Here's how the part is built. I have some questions about the finished solid (model axes, mm). A direction names the side the tool comes from. Round coordinates to 2 decimals unless told otherwise and drop trailing zeros. Loops run counter-clockwise (first coordinate to the right, second up) from the corner with the lowest first, then second, coordinate; pieces in that order, holes last. Notation, with made-up numbers: (-40, -21.75) - (-25, -21.75) arc R30 ccw to (-25, 10.25) - close; hole circle Ø11 at (-14, 7). An arc over 180 degrees is marked (long way). Answer as a JSON object with one key per item and string values. Group by question number.
1) I want a section at C-C, the plane x = 30. Please give me the cut outline in (y, z).
2) I want a section at D-D, the plane z = 46. Please give me the cut outline in (x, y), then the cut area to 3 significant figures.
3) I want a section at B-B, the plane y = 21.75. Please give me the cut outline in (x, z), then the cut area to 3 significant figures.
4) If I drill on line 1 along Z through (x, y) = (27.5, 21.75); line 2 along Z through (x, y) = (14.5, 7.75); line 3 along Z through (x, y) = (18.5, 21.75), over which ranges is the centre line in solid material (lowest first)? Write a range as [from, to].
5) I want a section at A-A, the plane y = 12. Give the number of separate pieces and of enclosed holes in the cut face, then the cut area to 3 significant figures.
6) If we mould it in two halves opening along Z, with no side actions, what happens to faces 1 (the face through (30, 12, 0)), 2 (the face through (21.584, 11.832, 27.473)), 3 (the face through (4.289, 11.832, 58.196))? For each: pulls with the +Z half, pulls with the -Z half, needs draft (parallel to the pull), parting line crosses it, or undercut.
7) Which directions (+Z, -Z, +X, -X, +Y, -Y) give clear straight access to the entire face, cutting with the end or side of a thin tool? Please do faces 4 (the face through (27.453, 11.832, 21.604)), 5 (the face through (29.8, 11.83, 17.78)), 6 (the face through (8.58, 11.83, 29.87)), 7 (the face through (2.96, 12.46, 48.47)).
8) Will these pins go through, and if not, where does the flat tip stop? P1, Ø8, axis at y = 5, z = 39, coming from the +X side; P2, Ø6.5, axis at x = 40.5, y = 17.5, coming from the +Z side; P3, Ø3, axis at y = 11, z = 22.5, coming from the +X side.
from build123d import *

# Parameters (mm, degrees)
F1_DEPTH = 24
F2_R     = 3.5
F3_DEPTH = 6
F4_R     = 3.5
F5_DEPTH = 6


# Not quite as in the source:
# - ends of sketch curves that miss each other by under 0.0002 mm in the source are joined


with BuildPart() as f1:
    # F0 (on Front) → F1 (new body)
    with BuildSketch(Plane.XZ):
        with BuildLine():
            Line((5.999886, 45.000227), (-0.000114, 45.000227))
            Line((-0.000114, 45.000227), (-0.000114, 0.000227))
            Line((-0.000114, 0.000227), (44.999886, 0.000227))
            Line((44.999886, 0.000227), (44.999886, 6.000227))
            Line((44.999886, 6.000227), (32.449634, 6.000227))
            Line((32.449634, 6.000227), (27.356487, 11.093373))
            ThreePointArc((27.356487, 11.093373), (26.477808, 13.214693), (27.3564876564, 15.3360133436))
            Line((27.3564876564, 15.3360133436), (32.306235, 20.285761))
            Line((32.306235, 20.285761), (28.523214, 24.068783))
            Line((28.523214, 24.068783), (26.755447, 22.301016))
            Line((26.755447, 22.301016), (28.16966, 20.886802))
            Line((28.16966, 20.886802), (23.960753, 16.677895))
            Line((23.960753, 16.677895), (16.64382, 21.098934))
            Line((16.64382, 21.098934), (18.091767, 22.546881))
            Line((18.091767, 22.546881), (16.677553, 23.961095))
            Line((16.677553, 23.961095), (20.88646, 28.170002))
            Line((20.88646, 28.170002), (22.300674, 26.755788))
            Line((22.300674, 26.755788), (24.068441, 28.523555))
            Line((24.068441, 28.523555), (20.28542, 32.306577))
            Line((20.28542, 32.306577), (15.335672, 27.356829))
            ThreePointArc((15.335672, 27.356829), (13.2143523536, 26.47815), (11.0930316564, 27.3568296564))
            Line((11.0930316564, 27.3568296564), (5.999886, 32.449975))
            Line((5.999886, 32.449975), (5.999886, 45.000227))
        make_face()
        with BuildLine():
            ThreePointArc((4.499886, 4.000227), (4.1463326094, 4.1466736094), (3.999886, 4.500227))
            Line((3.999886, 4.500227), (3.999886, 29.000227))
            ThreePointArc((3.999886, 29.000227), (4.3085446105, 29.4621669016), (4.8534398906, 29.3537798906))
            Line((4.8534398906, 29.3537798906), (13.567905, 20.639315))
            Line((13.567905, 20.639315), (11.243789, 18.315199))
            ThreePointArc((11.243789, 18.315199), (10.3880809238, 17.170688427), (9.8910739732, 15.8308650058))
            Line((9.8910739732, 15.8308650058), (11.753138, 13.968801))
            Line((11.753138, 13.968801), (12.364509, 14.132617))
            ThreePointArc((12.364509, 14.132617), (16.54708952, 16.547432386), (14.1322760675, 12.364850252))
            Line((14.1322760675, 12.364850252), (13.968459, 11.75348))
            Line((13.968459, 11.75348), (15.830523, 9.891416))
            ThreePointArc((15.830523, 9.891416), (17.1703461165, 10.3884227548), (18.3148569059, 11.2441310941))
            Line((18.3148569059, 11.2441310941), (20.638973, 13.568247))
            Line((20.638973, 13.568247), (29.353439, 4.853781))
            ThreePointArc((29.353439, 4.853781), (29.461825631, 4.3088849572), (28.999886, 4.000227))
            Line((28.999886, 4.000227), (4.499886, 4.000227))
        make_face(mode=Mode.SUBTRACT)
        with BuildLine():
            Line((3.999886, 29.000227), (3.999886, 4.500227))
            ThreePointArc((3.999886, 4.500227), (4.1463326094, 4.1466736094), (4.499886, 4.000227))
            Line((4.499886, 4.000227), (28.999886, 4.000227))
            ThreePointArc((28.999886, 4.000227), (29.461825631, 4.3088849572), (29.3534398906, 4.8537798906))
            Line((29.3534398906, 4.8537798906), (20.638973, 13.568247))
            Line((20.638973, 13.568247), (18.314857, 11.244131))
            ThreePointArc((18.314857, 11.244131), (17.1703461165, 10.3884227548), (15.8305230058, 9.8914159732))
            Line((15.8305230058, 9.8914159732), (13.968459, 11.75348))
            Line((13.968459, 11.75348), (14.132276, 12.36485))
            ThreePointArc((14.132276, 12.36485), (16.54708952, 16.547432386), (12.364508569, 14.1326168845))
            Line((12.364508569, 14.1326168845), (11.753138, 13.968801))
            Line((11.753138, 13.968801), (9.891074, 15.830865))
            ThreePointArc((9.891074, 15.830865), (10.3880809238, 17.170688427), (11.2437895941, 18.3151994059))
            Line((11.2437895941, 18.3151994059), (13.567905, 20.639315))
            Line((13.567905, 20.639315), (4.853439, 29.353781))
            ThreePointArc((4.853439, 29.353781), (4.3085446105, 29.4621669016), (3.999886, 29.000227))
        make_face()
        with BuildLine():
            ThreePointArc((5.999886, 54.000227), (4.2425266871, 58.2428676871), (-0.000114, 60.000227))
            Line((-0.000114, 60.000227), (-0.000114, 45.000227))
            Line((-0.000114, 45.000227), (5.999886, 45.000227))
            Line((5.999886, 45.000227), (5.999886, 54.000227))
        make_face()
        with BuildLine():
            Line((44.999886, 6.000227), (44.999886, 0.000227))
            Line((44.999886, 0.000227), (59.999886, 0.000227))
            ThreePointArc((59.999886, 0.000227), (58.2425266871, 4.2428676871), (53.999886, 6.000227))
            Line((53.999886, 6.000227), (44.999886, 6.000227))
        make_face()
    extrude(amount=-F1_DEPTH)

    # F2 (on face) → F3 (cut)
    with BuildSketch(Plane(origin=(-0.000114, 0, 0), x_dir=(0, -1, 0), z_dir=(-1, 0, 0))):
        with Locations((-12, 45.000227)):
            Circle(F2_R)
    extrude(amount=-F3_DEPTH, mode=Mode.SUBTRACT)

    # F4 (on face) → F5 (cut)
    with BuildSketch(Plane(origin=(0, 0, 0.000227), x_dir=(1, 0, 0), z_dir=(0, 0, -1))):
        with Locations((44.999886, -12)):
            Circle(F4_R)
    extrude(amount=-F5_DEPTH, mode=Mode.SUBTRACT)


solid = f1.part
Outcome:
{
 "1": {"outline": "(0, 0) - (24, 0) - (24, 8.45) - (0, 8.45) - close; (0, 17.98) - (24, 17.98) - (24, 22.59) - (0, 22.59) - close"},
 "2": {"outline": "(0, 0) - (6, 0) - (6, 8.65) - (0, 8.65) - close; (0, 15.35) - (6, 15.35) - (6, 24) - (0, 24) - close", "area": "104 mm^2"},
 "3": {"outline": "(0, 0) - (60, 0) arc R6 ccw to (54, 6) - (32.45, 6) - (27.36, 11.09) arc R3 cw to (27.36, 15.34) - (32.31, 20.29) - (28.52, 24.07) - (26.76, 22.3) - (28.17, 20.89) - (23.96, 16.68) - (16.64, 21.1) - (18.09, 22.55) - (16.68, 23.96) - (20.89, 28.17) - (22.3, 26.76) - (24.07, 28.52) - (20.29, 32.31) - (15.34, 27.36) arc R3 cw to (11.09, 27.36) - (6, 32.45) - (6, 54) arc R6 ccw to (0, 60) - close", "area": "1,110 mm^2"},
 "4": {"line 1": "[0, 10.95], [15.48, 20.22], [21.56, 23.05]", "line 2": "[0, 26.77]", "line 3": "[0, 19.98], [25.78, 30.52]"},
 "5": {"separate pieces": "3", "enclosed holes": "0", "area": "1,020 mm^2"},
 "6": {"face 1": "pulls with the -Z half", "face 2": "undercut", "face 3": "pulls with the +Z half"},
 "7": {"face 4": "+Y, -Y", "face 5": "+X, +Y, -Y", "face 6": "+Z, +Y, -Y", "face 7": "+X, -X"},
 "8": {"P1": "x = 6", "P2": "z = 6", "P3": "x = 31.59"}
}
